Could you check a few things on this model? Use its own coordinates, in mm. A direction names the side the tool comes from. Round coordinates to 2 decimals unless told otherwise and drop trailing zeros. Loops run counter-clockwise (first coordinate to the right, second up) from the corner with the lowest first, then second, coordinate; pieces in that order, holes last. Notation, with made-up numbers: M 45,27 L 89,27 A21 cw 89,43 Z; hole C 42.5,-32 d6. An arc over 180 degrees is marked long. One line per item, written item: value. Start each with the question number.
Q1. Imagine slicing it at B-B (y = -1.9). Please give me the cut outline in (x, z), then the cut area to 3 significant figures.
Q2. Which directions (+Z, -Z, +X, -X, +Y, -Y) give clear straight access to the entire face, cutting with the end or side of a thin tool? Please do faces 1 (the face through (-35, -2, -105.058)), 2 (the face through (-5.82, -2, -52)).
Q3. Thinking about a two-plate mould opening in X: for faces 3 (the face through (-55, 0, -50)), 4 (the face through (-64.558, -2, -50)), 5 (the face through (-21.695, -2, -49)), which applies, released by +X, released by -X, zero draft, split by the parting line, or undercut?
Q4. Imagine slicing it at A-A (z = -100.5). Please give me the cut outline in (x, y) (3 decimals).
Q5. Please list where these lines run through material, in increasing order: line 1 along Z through (x, y) = (-58, -1.05); line 2 along X through (y, z) = (-0.95, -97); line 3 along Z through (x, y) = (-56, -1.2).
Q6. Imagine slicing it at C-C (x = -35.5). Please give me the cut outline in (y, z) (3 decimals), then the cut area to 3 significant figures.
Q7. I'm going to push flat-ended pins straight in: pin 1 Ø8 at (x, z) = (-12.17, -54.26) entering from +Y; pin 2 Ø1.6 at (x, y) = (-40.5, -2.5) entering from +Z. Where does each tip first touch, or does it pass through?
from build123d import *

# Parameters (mm, degrees)
F0_W     = 3.175
F0_H     = 114.3
F0_R     = 2.54
F1_DEPTH = 3.175


with BuildPart() as f1:
    # F0 (on Front) → F1 (new body)
    with BuildSketch(Plane.XZ):
        with Locations((-50.270172, -47.908469)):
            Rectangle(F0_W, F0_H)
        Polygon((-21.695172, -105.058469), (-48.682672, -105.058469), (-51.857672, -105.058469), (-51.857672, 9.241531), (-64.557672, 9.241531), (-64.557672, -111.408469), (-5.820172, -111.408469), (-5.820172, 9.241531), (-18.520172, 9.241531), (-18.520172, -105.058469), align=None)
        with Locations((-58.207672, -86.008469)):
            Circle(F0_R, mode=Mode.SUBTRACT)
        with Locations((-58.207672, -54.258469)):
            Circle(F0_R, mode=Mode.SUBTRACT)
        with Locations((-12.170172, -86.008469)):
            Circle(F0_R, mode=Mode.SUBTRACT)
        with Locations((-12.170172, -54.258469)):
            Circle(F0_R, mode=Mode.SUBTRACT)
        with Locations((-58.207672, -22.508469)):
            Circle(F0_R, mode=Mode.SUBTRACT)
        with Locations((-12.170172, -22.508469)):
            Circle(F0_R, mode=Mode.SUBTRACT)
        with Locations((-20.107672, -47.908469)):
            Rectangle(F0_W, F0_H)
    extrude(amount=F1_DEPTH)


solid = f1.part
Report:
1. outline: M -64.56,-111.41 L -5.82,-111.41 L -5.82,9.24 L -21.7,9.24 L -21.7,-105.06 L -48.68,-105.06 L -48.68,9.24 L -64.56,9.24 Z; hole C -58.21,-86.01 d5.08; hole C -58.21,-54.26 d5.08; hole C -58.21,-22.51 d5.08; hole C -12.17,-86.01 d5.08; hole C -12.17,-54.26 d5.08; hole C -12.17,-22.51 d5.08
1. area: 3,880 mm²
2. face 1: +Z, +Y, -Y
2. face 2: +Z, -Z, +X, +Y, -Y
3. face 3: zero draft
3. face 4: released by -X
3. face 5: undercut
4. outline: M -64.558,-3.175 L -48.683,-3.175 L -48.683,0 L -64.558,0 Z; M -21.695,-3.175 L -5.82,-3.175 L -5.82,0 L -21.695,0 Z
5. line 1: z = -111.41 to -88.54, -83.48 to -56.79, -51.73 to -25.04, -19.98 to 9.24
5. line 2: x = -64.56 to -48.68, -21.7 to -5.82
5. line 3: z = -111.41 to -87.26, -84.75 to -55.51, -53 to -23.76, -21.25 to 9.24
6. outline: M -3.175,-111.408 L 0,-111.408 L 0,-105.058 L -3.175,-105.058 Z
6. area: 20.2 mm²
7. pin 1: stops at y = 0
7. pin 2: stops at z = -105.06
